Could you check a few things on this drawing? It's one solid part, dimensions in mm from its lowest x, y, z. Give positions to 0.01 mm unless a question says otherwise; leave off trailing zeros. Order: outer loops, then holes, each group sorted by start corner. A loop starts at its lowest first (then second) coordinate and runs counter-clockwise, first axis right, second up.
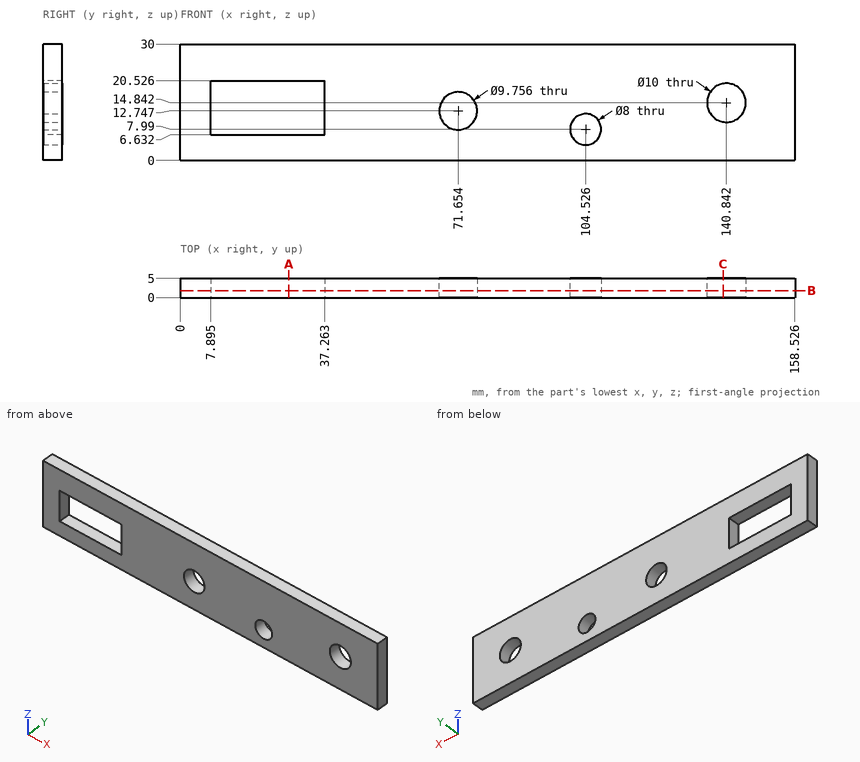
Item 1: Imagine slicing it at C-C on x = 140. List the corners of the cut face in (y, z) for me.
Findings:
outline: (0, 0) - (5, 0) - (5, 9.91) - (0, 9.91) - close; (0, 19.77) - (5, 19.77) - (5, 30) - (0, 30) - close
Item 2: Imagine slicing it at A-A on x = 28. List the corners of the cut face in (y, z) for me.
Findings:
outline: (0, 0) - (5, 0) - (5, 6.63) - (0, 6.63) - close; (0, 20.53) - (5, 20.53) - (5, 30) - (0, 30) - close
Item 3: Imagine slicing it at B-B on y = 1.8. List the corners of the cut face in (x, z) for me (1 decimal), then the cut area to 3 significant figures.
Findings:
outline: (0, 0) - (158.5, 0) - (158.5, 30) - (0, 30) - close; hole (7.9, 6.6) - (37.3, 6.6) - (37.3, 20.5) - (7.9, 20.5) - close; hole circle Ø9.8 at (71.7, 12.7); hole circle Ø8 at (104.5, 8); hole circle Ø10 at (140.8, 14.8)
area: 4,140 mm2
Item 4: Please list where these lines run through material, in increasing order: line 1 along Z through (x, y) = (11, 2.95); line 2 along X through (y, z) = (3.6, 13) (1 decimal); line 3 along X through (y, z) = (0.4, 12.25) (1 decimal).
Findings:
line 1: z = 0 to 6.63, 20.53 to 30
line 2: x = 0 to 7.9, 37.3 to 66.8, 76.5 to 136.2, 145.5 to 158.5
line 3: x = 0 to 7.9, 37.3 to 66.8, 76.5 to 136.6, 145.1 to 158.5
